Geometry check sheet. Reference: the model listing, model coordinates, mm. Face numbers are marked on the shaded views. A direction names the side the tool comes from. Give positions to 0.01 mm unless a question says otherwise; leave off trailing zeros. Write each loop counter-clockwise with the first axis right and the second up, starting at its lowest first coordinate (ties: lowest second). Pieces come first, ordered by that corner, then holes. Notation, with made-up numbers: M 69,48.25 L 75,48.25 A20 cw 75,82.25 Z; hole C 34.25,69.25 d7. An arc over 180 degrees is marked long. One line per item, written item: value. Start each with the question number.
1. Cross-section at D-D on x = 4.5. Record the cut outline in (y, z).
2. Cross-section at A-A on z = 0. Record the cut outline in (x, y).
3. Tool access check on the marked faces 1 and 2. Record the directions out of +Z, -Z, +X, -X, +Y, -Y that give a thin tool (end or side, any length) a straight path to the whole face; none if there is none.
4. Gauge pin test, flat ends, axial feed: pin 1 (2 mm diameter, centred on x = 1, z = -5.5, fed in from -Y); pin 2 (6 mm diameter, centred on x = -3.5, y = -6, fed in from -Z); pin 3 (12 mm diameter, centred on y = 3, z = 0, fed in from -X); pin 4 (1 mm diameter, centred on x = 0.5, z = 4, fed in from +Y). Record the tip position at first contact, or that the pin passes through.
5. Cross-section at C-C on x = -3. Record the cut outline in (y, z), then the cut area to 3 significant figures.
6. Scan lines: line 1 (Z direction, x = -1, y = 0); line 2 (X direction, y = -3, z = 10.5); line 3 (Z direction, x = 3, y = -3.5). Record each from-to range of solid material in increasing order.
7. Release check for a two-part mould opening along Z. For the marked faces 3, 4 and 5 record: pulls with the +Z half, pulls with the -Z half, needs draft (parallel to the pull), parting line crosses it, or undercut.
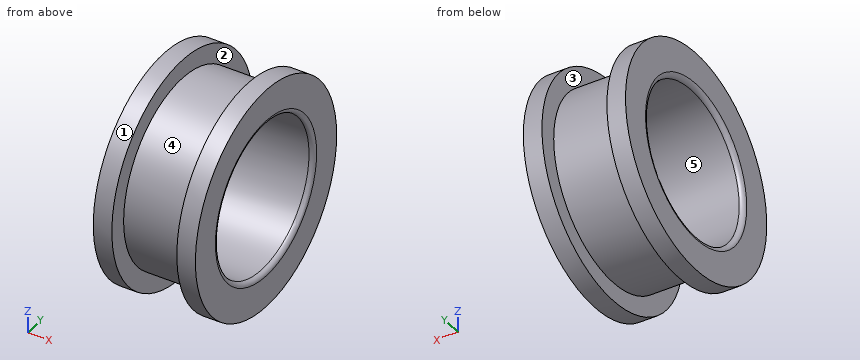
Autodesk Inventor part; units mm, degrees
ref_plane "YZ Plane" through (0, 0, 0) normal (1, 0, 0) x (0, 1, 0)
ref_plane "XZ Plane" through (0, 0, 0) normal (0, 1, 0) x (-1, 0, 0)
ref_plane "XY Plane" through (0, 0, 0) normal (0, 0, 1) x (1, 0, 0)
sketch "Sketch1" plane through (0, 0, 0) normal (0, 0, 1) x (1, 0, 0)
  line L0 (5.5, 8.1) -> (5.5, 12)
  line L1 (5.5, 12) -> (3.5, 12)
  line L2 (3.5, 12) -> (3.5, 10)
  line L3 (3.5, 10) -> (0, 10)
  line L4 (5.5, 8.1) -> (0, 8.1)
  line L5 (0, 8.1) -> (0, 10)
  line L6 (-2.3, 0) -> (6.8, 0)
  line L7 (0, 5.6) -> (0, 23.1)
  line L8 (0, 14.6) -> (0, 8.1)
  line L9 (0, 20.6) -> (0, 14.6)
  point P0 (0, 9.05)
  point P1 (-1, 12)
  point P2 (4.5, 12)
  dimension "d0" = 5.5
  dimension "d1" = 3.5
  dimension "d2" = 10
  dimension "d3" = 12
  dimension "d4" = 8.1
  dimension "d8" = 1
revolve "Revolution1" add sketch "Sketch1" angle 360 about axis through (-10, 0, 0) along (1, 0, 0)
mirror "Mirror2" about plane through (0, 0, 0) normal (1, 0, 0) of "Revolution1"
fillet "Fillet1" radius 0.5 2 edges at (5.5, -8.1, 0) (-5.5, -8.1, 0)
properties part number "Idler_Pulley_Overlay_3DPrint"
Report:
1. outline: C 0,0 d24; hole C 0,0 d16.2
2. outline: M -5.5,-12 L -3.5,-12 L -3.5,-10 L 3.5,-10 L 3.5,-12 L 5.5,-12 L 5.5,-8.6 A0.5 ccw 5,-8.1 L -5,-8.1 A0.5 ccw -5.5,-8.6 Z; M -5.5,8.6 A0.5 ccw -5,8.1 L 5,8.1 A0.5 ccw 5.5,8.6 L 5.5,12 L 3.5,12 L 3.5,10 L -3.5,10 L -3.5,12 L -5.5,12 Z
3. face 1: +X, -X
3. face 2: none
4. pin 1: stops at y = -8.93
4. pin 2: stops at z = -11.62
4. pin 3: stops at x = -5.5
4. pin 4: stops at y = 9.37
5. outline: C 0,0 d20; hole C 0,0 d16.2
5. area: 108 mm^2
6. line 1: z = -10 to -8.1, 8.1 to 10
6. line 2: x = -5.5 to -3.5, 3.5 to 5.5
6. line 3: z = -9.37 to -7.3, 7.3 to 9.37
7. face 3: needs draft
7. face 4: parting line crosses it
7. face 5: undercut
